Verification items for the finished model (mm, model axes). A direction names the side the tool comes from. Round coordinates to 2 decimals unless told otherwise and drop trailing zeros. Write each loop counter-clockwise with the first axis right and the second up, starting at its lowest first coordinate (ties: lowest second). Pieces come first, ordered by that corner, then holes. Notation, with made-up numbers: M -9.5,24 L 34.5,24 A20 cw 34.5,37 Z; hole C -8,3.25 d10. An arc over 180 degrees is marked long. One line per item, written item: value. Start each with the question number.
Item 1: Thickness scan on probe 1 along X at (y, z) = (19.5, -2); probe 2 along Z at (x, y) = (74.75, 12.5); probe 3 along Z at (x, y) = (21.1, 12.5). Record the ranges inside material, lowest first. Write a range as from..to.
Item 2: Gauge pin test, flat ends, axial feed: pin 1 (3 mm diameter, centred on x = 29, y = 15.5, fed in from +Z); pin 2 (2 mm diameter, centred on x = 16, y = 18, fed in from -Z); pin 3 (5 mm diameter, centred on y = 13, z = -4, fed in from +X); pin 4 (5 mm diameter, centred on y = 14, z = 15.5, fed in from +X). Record the tip position at first contact, or that the pin passes through.
Item 3: Section check B-B, the plane z = 10. Record the cut outline in (x, y), then the cut area to 3 significant figures.
Item 4: Section check D-D, the plane x = 98. Record the cut outline in (y, z), then the cut area to 3 significant figures.
Item 5: Section check C-C, the plane y = 23. Record the cut outline in (x, z).
Item 6: Draft check along Y on faces 4 (the face through (114, 12, 3)), 5 (the face through (22.54, 11.67, 12.62)), 6 (the face through (66.9, 12.32, 3.35)). Enter one of: +Y half, -Y half, draft (parallel to the pull), parting line (faces both ways), or undercut.
Item 7: Section check A-A, the plane x = 76.5. Record the cut outline in (y, z).
Item 8: Tool access check on faces 1 (the face through (112, 13, 13.349)), 2 (the face through (79.9, 13, -1)), 3 (the face through (20, 12, 6)). Record the directions out of +Z, -Z, +X, -X, +Y, -Y that give a thin tool (end or side, any length) a straight path to the whole face; none if there is none.
Autodesk Fusion 360 part; units mm, degrees
sketch "Sketch1" plane through (0, 0, 0) normal (0, 1, 0) x (1, 0, 0)
  line L0 (0, 0) -> (20, 0)
  line L1 (20, 0) -> (20, -20)
  line L2 (20, -20) -> (0, -20)
  line L3 (0, -20) -> (0, 0)
  line L4 (10, -20) -> (10, -25) construction
  line L5 (7, -25) -> (13, -25)
  line L6 (13, -25) -> (13, -14)
  line L7 (13, -14) -> (7, -14)
  line L8 (7, -14) -> (7, -25)
  line L9 (13, -25) -> (25, -25)
  line L10 (25, -25) -> (25, 0)
  line L11 (25, 0) -> (20, 0)
  dimension "d1" = 20
  dimension "d2" = 20
  dimension "d3" = 5
  dimension "d4" = 6
  dimension "d5" = 6
  dimension "d6" = 5
extrude "Extrude1" add sketch "Sketch1" along normal blind 25 contours L1 L2 L6 L9 L10 L11 | L2 L6 L7 L8 | L2 L5 L6 L8
hole "Hole3" at (20, 12.5, 10) direction (1, 0, 0) diameter 5.5 depth 11 tip angle 180
sketch "Sketch2" plane through (25, 0, 0) normal (1, 0, 0) x (0, 1, 0)
  line L0 (0, 25) -> (0, 0)
  line L1 (0, 0) -> (25, 0)
  line L2 (25, 0) -> (25, 25)
  line L3 (25, 25) -> (0, 25)
  arc A0 (25, 0) -> (0, 0) centre (12.5, -21.6506) ccw
  line L4 (0, 0) -> (0, -13)
  circle A1 centre (12.5, 10) radius 2.75
  line L5 (0, -13) -> (1.1286, -13)
  line L6 (1.1286, -13) -> (25, -13)
  line L7 (25, -13) -> (25, 0)
  dimension "d9" = 25
  dimension "d62" = 13
extrude "Extrude2" add sketch "Sketch2" along normal blind 85 and the other way blind 5 contours L1 A0 | L1 L4 L5 L6 L7
sketch "Sketch3" plane through (110, 0, 0) normal (1, 0, 0) x (0, 1, 0)
  arc A0 (25, 0) -> (0, 0) centre (12.5, -21.6506) ccw
  line L0 (0, 0) -> (0, -13)
  line L1 (25, -13) -> (25, 0)
  line L2 (12.5, -16.6506) -> (12.5, 13.3494) construction
  line L3 (25, 13.3494) -> (25, 0)
  line L4 (25, 13.3494) -> (0, 13.3494)
  line L5 (0, 13.3494) -> (0, 0)
  line L6 (0, -13) -> (25, -13)
  dimension "d12" = 10
  dimension "d13" = 25
extrude "Extrude3" add sketch "Sketch3" along normal blind 4
chamfer "Chamfer1" distance 3 angle 45 2 edges at (7, 12.5, 25) (25, 12.5, 25)
chamfer "Chamfer2" distance 3 angle 45 2 edges at (10, 0, 14) (10, 25, 14)
chamfer "Chamfer5" distance 7.5 angle 45 2 edges at (112, 0, 13.3494) (112, 25, 13.3494)
chamfer "Chamfer6" distance 5 angle 45 2 edges at (20, 12.5, -13) (114, 12.5, -13)
sketch "Sketch4" plane through (0, 0, 25) normal (0, 0, 1) x (-1, 0, 0)
  line L0 (-25, -25) -> (-25, 0)
  line L1 (-25, 0) -> (-110, 0)
  line L2 (-110, 0) -> (-110, -25)
  line L3 (-110, -25) -> (-25, -25)
  line L4 (-67.5, -25) -> (-67.5, 0) construction
  line L5 (-49.5, -25) -> (-85.5, -25)
  line L6 (-85.5, -25) -> (-85.5, 0)
  line L7 (-85.5, 0) -> (-49.5, 0)
  line L8 (-49.5, 0) -> (-49.5, -25)
  line L9 (-55.1, -25) -> (-79.9, -25)
  line L10 (-79.9, -25) -> (-79.9, 0)
  line L11 (-79.9, 0) -> (-55.1, 0)
  line L12 (-55.1, 0) -> (-55.1, -25)
  line L13 (-49.5, -12.5) -> (-85.5, -12.5) construction
  line L14 (-49.5, -20.75) -> (-85.5, -20.75)
  line L15 (-85.5, -20.75) -> (-85.5, -4.25)
  line L16 (-85.5, -4.25) -> (-49.5, -4.25)
  line L17 (-49.5, -4.25) -> (-49.5, -20.75)
  line L18 (-64.5, -20.75) -> (-70.5, -20.75)
  line L19 (-70.5, -20.75) -> (-70.5, -4.25)
  line L20 (-70.5, -4.25) -> (-64.5, -4.25)
  line L21 (-64.5, -4.25) -> (-64.5, -20.75)
  line L22 (-22, 0) -> (-22, -25)
  line L23 (-22, -25) -> (-10, -25)
  line L24 (-10, -25) -> (-10, 0)
  line L25 (-10, 0) -> (-22, 0)
  dimension "d22" = 36
  dimension "d23" = 5.6
  dimension "d24" = 20
  dimension "d25" = 16.5
  dimension "d29" = 21.5
  dimension "d31" = 6
extrude "Extrude4" cut sketch "Sketch4" against normal blind 27 from surface at -5 contours L8 L12 L14 L16 L17 | L6 L10 L14 L15 L16
hole "Hole1" at (114, 12.5, -4.3253) direction (-1, 0, 0) diameter 5 depth 100 tip angle 118 counterbore diameter 10 counterbore depth 22
hole "Hole2" at (20, 12.5, -4.3253) direction (1, 0, 0) diameter 10 depth 23 tip angle 118
equation "d62 = 5 mm + 4 mm + 4 mm"
Response values:
1. probe 1: x = 20..49.5, 55.1..79.9, 85.5..114
1. probe 2: z = -13..-6.83, -1.83..3.35
1. probe 3: z = 0.67..7.25, 12.75..25
2. pin 1: stops at z = 3.3
2. pin 2: stops at z = 20
2. pin 3: stops at x = 92
2. pin 4: stops at x = 114
3. outline: M 20,0 L 25,0 L 25,9.75 L 20,9.75 Z; M 20,15.25 L 25,15.25 L 25,25 L 20,25 Z; M 110,4.15 L 114,4.15 L 114,20.85 L 110,20.85 Z
3. area: 164 mm2
4. outline: M 0,-13 L 25,-13 L 25,0 A25 ccw 0,0 Z; hole C 12.5,-4.33 d10
4. area: 303 mm2
5. outline: M 7,15 L 13,15 L 13,20 L 20,20 L 20,-8 L 25,-13 L 109,-13 L 114,-8 L 114,7.85 L 110,7.85 L 110,1.04 L 25,1.04 L 25,22 L 22,25 L 10,25 L 7,22 Z
6. face 4: draft
6. face 5: undercut
6. face 6: parting line
7. outline: M 0,-13 L 25,-13 L 25,0 A25 ccw 0,0 Z; hole C 12.5,-4.33 d5
8. face 1: +Z, +X, +Y, -Y
8. face 2: +Z
8. face 3: -Z, +Y, -Y
